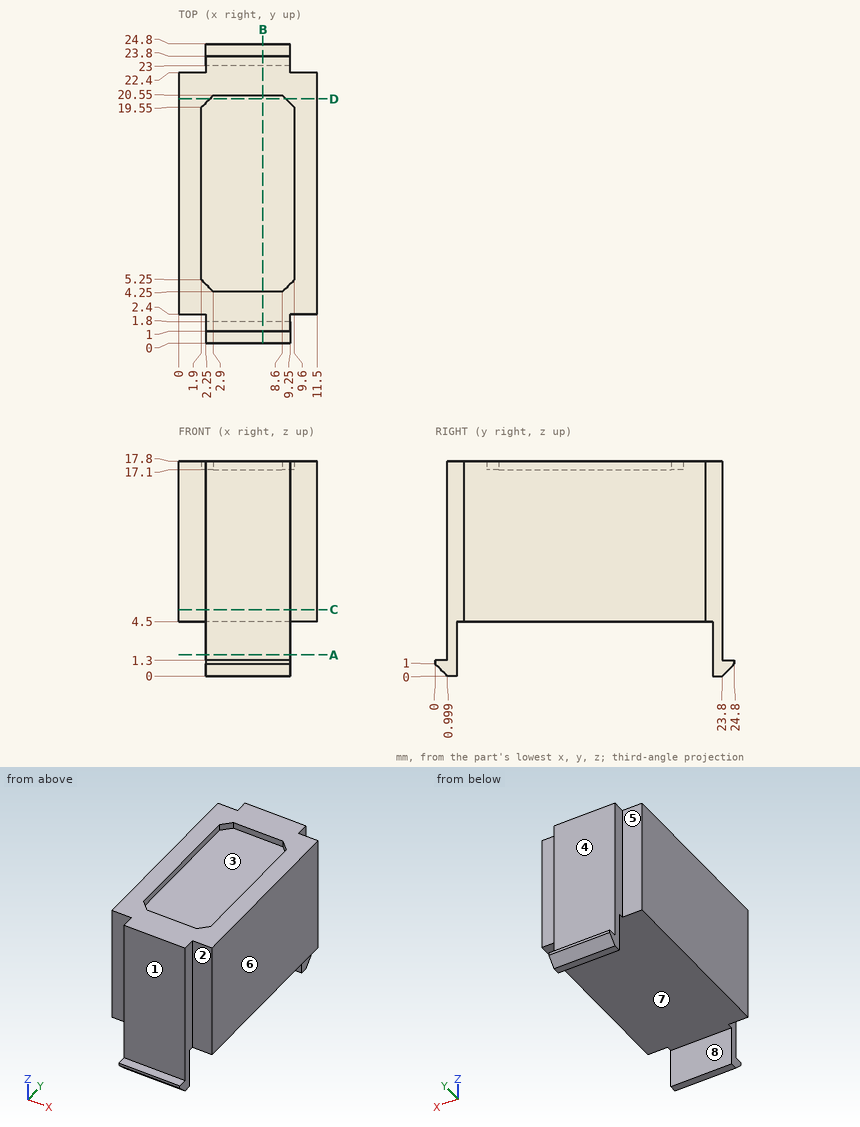
Could you check a few things on this drawing? It's one solid part, dimensions in mm from its lowest x, y, z. A direction names the side the tool comes from. Coordinates: 2 decimals unless noted, no trailing zeros. Order: outer loops, then holes, each group sorted by start corner. A loop starts at its lowest first (then second) coordinate and runs counter-clockwise, first axis right, second up. Notation, with made-up numbers: (-32.5, 1) - (-21.5, 1) arc R21 ccw to (-21.5, 32) - close; hole circle Ø1 at (78.5, 66). An arc over 180 degrees is marked (long way). Answer as a JSON object with one key per item and string values. Group by question number.
Q1. On a 3-axis mill with a long thin cutter (end or side, diameter ignored), from which of +Z, -Z, +X, -X, +Y, -Y can I reach the whole of each face in a straight line? I mean the marked faces 1, 2, 3 and 4. Say none if no direction works.
Q2. We'd pull the mould along Y, two halves only. Please class the marked faces 5, 6, 7 and 8: +Y half, -Y half, draft (parallel to the pull), parting line (faces both ways), or undercut.
Q3. Imagine slicing it at B-B (x = 7). Please give me the cut outline in (y, z).
Q4. Imagine slicing it at A-A (z = 1.75). Please give me the cut outline in (x, y), and give its area (3 significant figures).
Q5. Imagine slicing it at D-D (y = 20.25). Please give me the cut outline in (x, z).
Q6. I need wall thicknesses on line 1 (Y direction, x = 6, z = 1.75); line 2 (Y direction, x = 5.75, z = 8.5); line 3 (X direction, y = 1.5, z = 15.75). Which ranges of each line are inside material? Lowest first, please. Write a range as from..to.
Q7. Will these pins go through, and if not, where does the flat tip stop? P1, Ø3, axis at x = 7, z = 13, coming from the +Y side; P2, Ø1.3, axis at x = 4, z = 3, coming from the -Y side; P3, Ø1, axis at x = 7.5, y = 4, coming from the -Z side.
Q8. Imagine slicing it at C-C (z = 5.5). Please give me the cut outline in (x, y), and give its area (3 significant figures).
Determined:
{
 "1": {"face 1": "+Z, +X, -X, -Y", "face 2": "+Z, -Z, +X, -Y", "face 3": "+Z", "face 4": "+Z, +X, -X, +Y"},
 "2": {"face 5": "+Y half", "face 6": "draft", "face 7": "undercut", "face 8": "undercut"},
 "3": {"outline": "(0, 1) - (1, 0) - (1.8, 0) - (1.8, 4.5) - (23, 4.5) - (23, 0) - (23.8, 0) - (24.8, 1) - (24.8, 1.3) - (23.8, 1.3) - (23.8, 17.8) - (20.55, 17.8) - (20.55, 17.1) - (4.25, 17.1) - (4.25, 17.8) - (1, 17.8) - (1, 1.3) - (0, 1.3) - close"},
 "4": {"outline": "(2.25, 1) - (9.25, 1) - (9.25, 1.8) - (2.25, 1.8) - close; (2.25, 23) - (9.25, 23) - (9.25, 23.8) - (2.25, 23.8) - close", "area": "11.2 mm2"},
 "5": {"outline": "(0, 4.5) - (11.5, 4.5) - (11.5, 17.8) - (8.9, 17.8) - (8.9, 17.1) - (2.6, 17.1) - (2.6, 17.8) - (0, 17.8) - close"},
 "6": {"line 1": "y = 1..1.8, 23..23.8", "line 2": "y = 1..23.8", "line 3": "x = 2.25..9.25"},
 "7": {"P1": "stops at y = 23.8", "P2": "stops at y = 1", "P3": "stops at z = 4.5"},
 "8": {"outline": "(0, 2.4) - (2.25, 2.4) - (2.25, 1) - (9.25, 1) - (9.25, 2.4) - (11.5, 2.4) - (11.5, 22.4) - (9.25, 22.4) - (9.25, 23.8) - (2.25, 23.8) - (2.25, 22.4) - (0, 22.4) - close", "area": "250 mm2"}
}
